Read the model definition and answer for the solid it produces. Units are mm, in the model's axes. A direction names the side the tool comes from. Give positions to 0.01 mm unless a question says otherwise; leave off trailing zeros. Order: outer loops, then holes, each group sorted by start corner. A loop starts at its lowest first (then second) coordinate and runs counter-clockwise, first axis right, second up. Notation, with made-up numbers: (60, 78) - (78, 78) arc R16 cw to (78, 89) - close; hole circle Ø5 at (51, -21). An arc over 180 degrees is marked (long way). Return JSON: item names as keys, results as strings.
```python
from build123d import *

# Parameters (mm, degrees)
BOSS_EXTRUDE1_DEPTH = 401.5
FILLET2_R           = 15
FILLET4_R           = 22


with BuildPart() as part:
    # Sketch1 → Boss-Extrude1 (new body)
    with BuildSketch(Plane.XY):
        Polygon((-95.35, 84.15), (-95.35, -76.3), (95.35, -76.3), (95.35, 84.15), (103.2, 84.15), (103.2, -84.15), (-103.2, -84.15), (-103.2, 84.15), align=None)
    extrude(amount=BOSS_EXTRUDE1_DEPTH)

    # Fillet2
    fillet2_edges = [part.edges().sort_by_distance(p)[0] for p in [
        (-95.35, -76.3, 200.75),
        (95.35, -76.3, 200.75),
    ]]
    fillet(fillet2_edges, radius=FILLET2_R)

    # Fillet4
    fillet4_edges = [part.edges().sort_by_distance(p)[0] for p in [
        (103.2, -84.15, 200.75),
        (-103.2, -84.15, 200.75),
    ]]
    fillet(fillet4_edges, radius=FILLET4_R)


solid = part.part
```
Q1. A cutting plane is placed at C-C (y = 27.5). Write down the section's boundary in (x, z), and give its area (3 significant figures).
Values:
{"outline": "(-103.2, 0) - (-95.35, 0) - (-95.35, 401.5) - (-103.2, 401.5) - close; (95.35, 0) - (103.2, 0) - (103.2, 401.5) - (95.35, 401.5) - close", "area": "6,300 mm²"}
Q2. Consider L1, parallel to X at y = 41, z = 187; L2, parallel to Y at x = -45.5, z = 53.5; L3, parallel to Y at x = -90, z = 351.5. Determine where each line is inside the solid, lowest interval first.
Values:
{"L1": "x = -103.2 to -95.35, 95.35 to 103.2", "L2": "y = -84.15 to -76.3", "L3": "y = -82.31 to -72.78"}
Q3. A cutting plane is placed at A-A (y = -72). Write down the section's boundary in (x, z), and give its area (3 significant figures).
Values:
{"outline": "(-100.87, 0) - (-90.86, 0) - (-90.86, 401.5) - (-100.87, 401.5) - close; (90.86, 0) - (100.87, 0) - (100.87, 401.5) - (90.86, 401.5) - close", "area": "8,040 mm²"}
Q4. Determine the mould class of faces 3 (the flat face through (0, -81, 401.5)), 4 (the cylindrical face through (-96.93, -77.53, 203.56)), 5 (the flat face through (95.35, 10, 198)), 6 (the flat face through (-1, -76.3, 198)) for opening direction X: released by +X, released by -X, zero draft, split by the parting line, or undercut.
Values:
{"face 3": "zero draft", "face 4": "released by -X", "face 5": "undercut", "face 6": "undercut"}
Q5. A cutting plane is placed at B-B (z = 61.5). Write down the section's boundary in (x, y).
Values:
{"outline": "(-103.2, -62.15) arc R22 ccw to (-81.2, -84.15) - (81.2, -84.15) arc R22 ccw to (103.2, -62.15) - (103.2, 84.15) - (95.35, 84.15) - (95.35, -61.3) arc R15 cw to (80.35, -76.3) - (-80.35, -76.3) arc R15 cw to (-95.35, -61.3) - (-95.35, 84.15) - (-103.2, 84.15) - close"}
Q6. Given pin 1 (1.5 mm diameter, centred on x = -55.5, z = 210.5, fed in from +Y), flat-ended and moving along its own axis, determine where the tip first touches the part or whether it passes through.
Values:
{"pin 1": "stops at y = -76.3"}
Q7. A cutting plane is placed at D-D (x = -14). Write down the section's boundary in (y, z), and give its area (3 significant figures).
Values:
{"outline": "(-84.15, 0) - (-76.3, 0) - (-76.3, 401.5) - (-84.15, 401.5) - close", "area": "3,150 mm²"}
Q8. For faces 1 (the flat face through (-95.35, 12, 198)), 2 (the flat face through (103.2, 12, 198)), determine the directions among +Z, -Z, +X, -X, +Y, -Y from which every point of the face is accessible in a straight line to the end or side of a thin tool.
Values:
{"face 1": "+Z, -Z, +Y", "face 2": "+Z, -Z, +X, +Y, -Y"}
